Read the model definition and answer for the solid it produces. Units are mm, in the model's axes. A direction names the side the tool comes from. Round coordinates to 2 decimals unless told otherwise and drop trailing zeros. Loops run counter-clockwise (first coordinate to the right, second up) from the corner with the lowest first, then second, coordinate; pieces in that order, holes last. Notation, with made-up numbers: M 81.25,34 L 130.25,34 A33 cw 130.25,70 Z; hole C 89.5,77.25 d8. An arc over 180 degrees is marked long. Write each question's results on one line, items separated by ' | '.
```python
from build123d import *

# Parameters (mm, degrees)
SKETCH_1_W      = 45
SKETCH_1_H      = 50
SKETCH_1_R      = 2.15
SKETCH_1_W_2    = 25
SKETCH_1_H_2    = 30
EXTRUDE_1_DEPTH = 5
FILLET_1_R      = 2
FILLET_2_R      = 3


with BuildPart() as part:
    # ｽｹｯﾁ1 → ﾎﾞｽ - 押し出し1 (new body)
    with BuildSketch(Plane.XY):
        with Locations((22.5, 25)):
            Rectangle(SKETCH_1_W, SKETCH_1_H)
        with Locations((5.5, 5)):
            Circle(SKETCH_1_R, mode=Mode.SUBTRACT)
        with Locations(Location((5.5, 45, 0), (0, 0, 180))):
            Circle(SKETCH_1_R, mode=Mode.SUBTRACT)
        with Locations(Location((39.5, 5, 0), (0, 0, 180))):
            Circle(SKETCH_1_R, mode=Mode.SUBTRACT)
        with Locations((39.5, 45)):
            Circle(SKETCH_1_R, mode=Mode.SUBTRACT)
        with Locations((22.5, 25)):
            Rectangle(SKETCH_1_W_2, SKETCH_1_H_2, mode=Mode.SUBTRACT)
    extrude(amount=EXTRUDE_1_DEPTH)

    # ﾌｨﾚｯﾄ1
    fillet_1_edges = [part.edges().sort_by_distance(p)[0] for p in [
        (0, 50, 2.5),
        (45, 50, 2.5),
        (45, 0, 2.5),
        (0, 0, 2.5),
    ]]
    fillet(fillet_1_edges, radius=FILLET_1_R)

    # ﾌｨﾚｯﾄ2
    fillet_2_edges = [part.edges().sort_by_distance(p)[0] for p in [
        (35, 10, 2.5),
        (35, 40, 2.5),
        (10, 40, 2.5),
        (10, 10, 2.5),
    ]]
    fillet(fillet_2_edges, radius=FILLET_2_R)


solid = part.part
```
1. Find the intervals of material crossed by L1, parallel to Y at x = 39.5, z = 2.75; L2, parallel to Y at x = 19, z = 1.05; L3, parallel to X at y = 14, z = 2.85, in increasing order.
Completed:
L1: y = 0 to 2.85, 7.15 to 42.85, 47.15 to 50 | L2: y = 0 to 10, 40 to 50 | L3: x = 0 to 10, 35 to 45
2. Find section C-C, the plane x = 5.5. Give the vertices of the cut face in (y, z).
Completed:
outline: M 0,0 L 2.85,0 L 2.85,5 L 0,5 Z; M 7.15,0 L 42.85,0 L 42.85,5 L 7.15,5 Z; M 47.15,0 L 50,0 L 50,5 L 47.15,5 Z
3. Find section B-B, the plane z = 1.35. Give the vertices of the cut face in (x, y), then the cut area to 3 significant figures.
Completed:
outline: M 0,2 A2 ccw 2,0 L 43,0 A2 ccw 45,2 L 45,48 A2 ccw 43,50 L 2,50 A2 ccw 0,48 Z; hole C 5.5,5 d4.3; hole C 5.5,45 d4.3; hole M 10,13 A3 ccw 13,10 L 32,10 A3 ccw 35,13 L 35,37 A3 ccw 32,40 L 13,40 A3 ccw 10,37 Z; hole C 39.5,5 d4.3; hole C 39.5,45 d4.3 | area: 1,450 mm2
4. Find section D-D, the plane x = 14.5. Give the vertices of the cut face in (y, z), then the cut area to 3 significant figures.
Completed:
outline: M 0,0 L 10,0 L 10,5 L 0,5 Z; M 40,0 L 50,0 L 50,5 L 40,5 Z | area: 100 mm2
5. Find section A-A, the plane y = 5. Give the vertices of the cut face in (x, z).
Completed:
outline: M 0,0 L 3.35,0 L 3.35,5 L 0,5 Z; M 7.65,0 L 37.35,0 L 37.35,5 L 7.65,5 Z; M 41.65,0 L 45,0 L 45,5 L 41.65,5 Z
6. Given P1, Ø5.5, axis at x = 39.5, y = 5, coming from the +Z side; P2, Ø4, axis at x = 5.5, y = 45, coming from the +Z side, each flat-ended and moving along its own axis, determine where each tip first touches the part or whether it passes through.
Completed:
P1: stops at z = 5 | P2: passes through
7. Which of the six approach directions +Z, -Z, +X, -X, +Y, -Y give full straight-line access (tool end or side, diameter ignored) to faces 4 (the face through (10, 25, 2)), 5 (the face through (44.4, 0.57, 2.54))?
Completed:
face 4: +Z, -Z | face 5: +Z, -Z, +X, -Y
8. Determine the mould class of faces 1 (the face through (7, 25, 5)), 2 (the face through (0.57, 49.4, 2.54)), 3 (the face through (37.45, 4.35, 2.46)) for opening direction X: released by +X, released by -X, zero draft, split by the parting line, or undercut.
Completed:
face 1: zero draft | face 2: released by -X | face 3: undercut
